Model file for the job. Use its own axes, mm. Give positions to 0.01 mm unless a question says otherwise; leave off trailing zeros. Write each loop counter-clockwise with the first axis right and the second up, starting at its lowest first coordinate (ties: lowest second). Pieces come first, ordered by that corner, then holes.
```python
from build123d import *

# Parameters (mm, degrees)
PAD_DEPTH = 3


with BuildPart() as part:
    # Sketch → Pad (new body)
    with BuildSketch(Plane.XY):
        Polygon((0, 0), (0, 17), (34.5, 17), (34.5, 8.5), (37.5, 8.5), (37.5, 17), (65.5, 17), (65.5, 8.5), (68.5, 8.5), (68.5, 17), (96.5, 17), (96.5, 8.5), (99.5, 8.5), (99.5, 17), (127.5, 17), (127.5, 8.5), (130.5, 8.5), (130.5, 17), (158.5, 17), (158.5, 8.5), (161.5, 8.5), (161.5, 17), (189.5, 17), (189.5, 8.5), (192.5, 8.5), (192.5, 17), (220.5, 17), (220.5, 8.5), (223.5, 8.5), (223.5, 17), (251.5, 17), (251.5, 8.5), (254.5, 8.5), (254.5, 17), (282.5, 17), (282.5, 8.5), (285.5, 8.5), (285.5, 17), (313.5, 17), (313.5, 8.5), (316.5, 8.5), (316.5, 17), (344.5, 17), (344.5, 8.5), (347.5, 8.5), (347.5, 17), (375.5, 17), (375.5, 8.5), (378.5, 8.5), (378.5, 17), (406.5, 17), (406.5, 8.5), (409.5, 8.5), (409.5, 17), (437.5, 17), (437.5, 8.5), (440.5, 8.5), (440.5, 17), (468.5, 17), (468.5, 8.5), (471.5, 8.5), (471.5, 17), (499.5, 17), (499.5, 8.5), (502.5, 8.5), (502.5, 17), (530.5, 17), (530.5, 8.5), (533.5, 8.5), (533.5, 17), (567.5, 17), (567.5, 0), (493.5, 0), (493.5, 2), (446.5, 2), (446.5, 0), (400.5, 0), (400.5, 2), (353.5, 2), (353.5, 0), (307.5, 0), (307.5, 2), (260.5, 2), (260.5, 0), (214.5, 0), (214.5, 2), (167.5, 2), (167.5, 0), (121.5, 0), (121.5, 2), (74.5, 2), (74.5, 0), align=None)
    extrude(amount=PAD_DEPTH)


solid = part.part
```
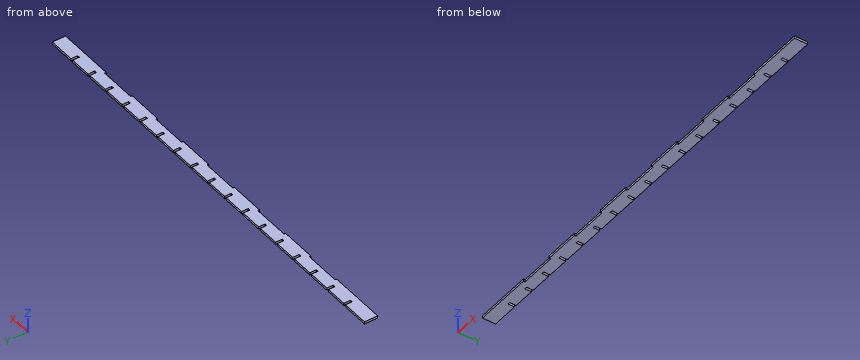
1. Pin check, flat tips, straight feed: P1, Ø0.9, axis at x = 501.5, z = 1.5, coming from the +Y side; P2, Ø1, axis at y = 1, z = 2, coming from the -X side; P3, Ø0.9, axis at x = 97, z = 1, coming from the -Y side. Stop position of each tip, or through.
Calculated:
P1: stops at y = 8.5
P2: stops at x = 0
P3: stops at y = 2
2. Probe probe 1 along Y at (x, z) = (270, 1.4); probe 2 along Y at (x, z) = (253, 1.45). List the from-to ranges inside material, lowest first.
Calculated:
probe 1: y = 2 to 17
probe 2: y = 0 to 8.5
3. Slice it at A-A, the plane y = 14. State how many separate pieces and enclosed holes the cut face has, and give its area (3 significant figures).
Calculated:
separate pieces: 18
enclosed holes: 0
area: 1,550 mm2
4. Slice it at B-B, the plane x = 111.5. Write the cut outline in (y, z).
Calculated:
outline: (2, 0) - (17, 0) - (17, 3) - (2, 3) - close
